Geometry: see drawing. Coordinates: mm, zero at the bounding-box minimum. A direction names the side the tool comes from. Round coordinates to 2 decimals unless told otherwise and drop trailing zeros. Write each loop counter-clockwise with the first axis right and the second up, starting at its lowest first coordinate (ties: lowest second). Pieces come first, ordered by that corner, then holes. Notation, with made-up numbers: (5, 55.5) - (62, 55.5) arc R15 ccw to (62, 64.5) - close; hole circle Ø9 at (-7.75, 48.5). An arc over 180 degrees is marked (long way). One line per item, written item: value. Start each with the question number.
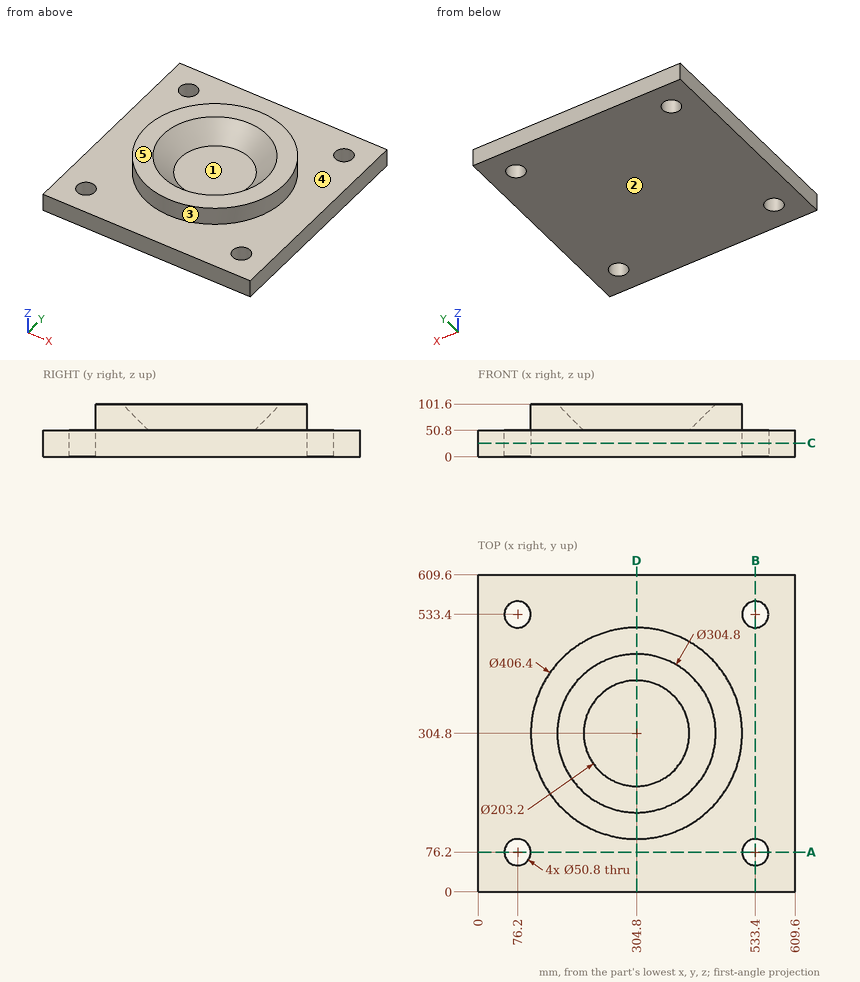
Q1. Contact query for flat-ended pins moving along their axis: pin 1 Ø8 at (x, y) = (395.5, 229.5) entering from +Z; pin 2 Ø2 at (x, z) = (192, 58.5) entering from -Y; pin 3 Ø4 at (x, z) = (127, 40) entering from -Y; pin 4 Ø8 at (y, z) = (224.5, 70) entering from -X. Output: stop coordinate, or through.
Q2. Pull-direction query (Y, two-part tool) for the marked faces 1, 2 and 3; classes: pulls with the +Y half, pulls with the -Y half, needs draft (parallel to the pull), parting line crosses it, or undercut.
Q3. Cut plane C-C, the plane z = 26.5. Output: boundary loops of the cut face in (x, y), and give its area (3 significant figures).
Q4. Access query for the marked faces 4 and 5. Directions: +Z, -Z, +X, -X, +Y, -Y. A direction counts if a zero-diameter tool reaches every point of the face in a straight line with its end or side. Return the directions, or none.
Q5. Cut plane A-A, the plane y = 76.2. Output: boundary loops of the cut face in (x, z).
Q6. Material intervals for probe 1 along Y at (x, z) = (76.2, 16); probe 2 along X at (y, z) = (540.5, 15.5), sorted ascending. Write a range as from..to.
Q7. Cut plane D-D, the plane x = 304.8. Output: boundary loops of the cut face in (y, z), and give its area (3 significant figures).
A:
1. pin 1: stops at z = 71.08
1. pin 2: stops at y = 135.12
1. pin 3: stops at y = 0
1. pin 4: stops at x = 116.47
2. face 1: undercut
2. face 2: needs draft
2. face 3: parting line crosses it
3. outline: (0, 0) - (609.6, 0) - (609.6, 609.6) - (0, 609.6) - close; hole circle Ø50.8 at (76.2, 76.2); hole circle Ø50.8 at (76.2, 533.4); hole circle Ø50.8 at (533.4, 76.2); hole circle Ø50.8 at (533.4, 533.4)
3. area: 364,000 mm²
4. face 4: +Z
4. face 5: +Z, +X, -X, +Y, -Y
5. outline: (0, 0) - (50.8, 0) - (50.8, 50.8) - (0, 50.8) - close; (101.6, 0) - (508, 0) - (508, 50.8) - (101.6, 50.8) - close; (558.8, 0) - (609.6, 0) - (609.6, 50.8) - (558.8, 50.8) - close
6. probe 1: y = 0..50.8, 101.6..508, 558.8..609.6
6. probe 2: x = 0..51.81, 100.59..509.01, 557.79..609.6
7. outline: (0, 0) - (609.6, 0) - (609.6, 50.8) - (508, 50.8) - (508, 101.6) - (457.2, 101.6) - (406.4, 50.8) - (203.2, 50.8) - (152.4, 101.6) - (101.6, 101.6) - (101.6, 50.8) - (0, 50.8) - close
7. area: 38,700 mm²
